Source: CAD feature listing. Evaluate the final solid. Frame: model axes, mm. Give positions to 0.01 mm unless a question says otherwise; leave off trailing zeros. Order: outer loops, then holes, each group sorted by start corner. A loop starts at its lowest first (then second) coordinate and runs counter-clockwise, first axis right, second up. Notation, with made-up numbers: (-31.5, -24) -> (2.5, -24) arc R17 cw to (2.5, -2) -> close; hole circle Ø10 at (2, -25). An arc over 180 degrees is marked (long way). Use CSV: the item, a comma, the result in double quotes.
```python
from build123d import *

# Parameters (mm, degrees)
SKETCH1_W           = 21
SKETCH1_H           = 9
BOSS_EXTRUDE1_DEPTH = 3


with BuildPart() as part:
    # Sketch1 → Boss-Extrude1 (new body)
    with BuildSketch(Plane.XY):
        Polygon((178.5, 24), (181.5, 24), (181.5, 27), (202.5, 27), (202.5, 24), (205.5, 24), (205.5, 27), (210, 27), (210, 28.5), (213, 28.5), (213, 30), (205.5, 30), (205.5, 39), (210, 39), (210, 40.5), (213, 40.5), (213, 42), (6, 42), (6, 40.5), (3, 40.5), (3, 39), (10.5, 39), (10.5, 30), (6, 30), (6, 28.5), (3, 28.5), (3, 27), (10.5, 27), (10.5, 24), (13.5, 24), (13.5, 27), (34.5, 27), (34.5, 24), (37.5, 24), (37.5, 27), (58.5, 27), (58.5, 24), (61.5, 24), (61.5, 27), (82.5, 27), (82.5, 24), (85.5, 24), (85.5, 27), (106.5, 27), (106.5, 24), (109.5, 24), (109.5, 27), (130.5, 27), (130.5, 24), (133.5, 24), (133.5, 27), (154.5, 27), (154.5, 24), (157.5, 24), (157.5, 27), (178.5, 27), align=None)
        with Locations((192, 34.5)):
            Rectangle(SKETCH1_W, SKETCH1_H, mode=Mode.SUBTRACT)
        with Locations((168, 34.5)):
            Rectangle(SKETCH1_W, SKETCH1_H, mode=Mode.SUBTRACT)
        with Locations((144, 34.5)):
            Rectangle(SKETCH1_W, SKETCH1_H, mode=Mode.SUBTRACT)
        with Locations((120, 34.5)):
            Rectangle(SKETCH1_W, SKETCH1_H, mode=Mode.SUBTRACT)
        with Locations((96, 34.5)):
            Rectangle(SKETCH1_W, SKETCH1_H, mode=Mode.SUBTRACT)
        with Locations((72, 34.5)):
            Rectangle(SKETCH1_W, SKETCH1_H, mode=Mode.SUBTRACT)
        with Locations((48, 34.5)):
            Rectangle(SKETCH1_W, SKETCH1_H, mode=Mode.SUBTRACT)
        with Locations((24, 34.5)):
            Rectangle(SKETCH1_W, SKETCH1_H, mode=Mode.SUBTRACT)
    extrude(amount=BOSS_EXTRUDE1_DEPTH)


solid = part.part
```
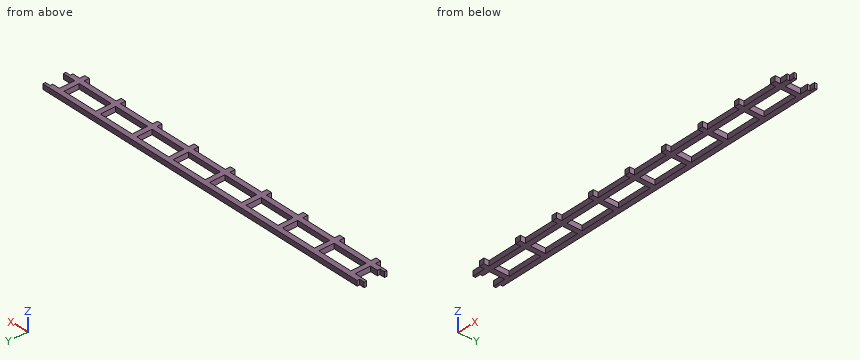
1. Ray query, line 1 along Y through (x, z) = (152, 0.65); line 2 along X through (y, z) = (39.5, 0.95); line 3 along X through (y, z) = (41.25, 2.3). Return the intervals inside material, ascending.
Answer below:
line 1,"y = 27 to 30, 39 to 42"
line 2,"x = 3 to 210"
line 3,"x = 6 to 213"
2. Pin query (flat end, axial travel): P1, Ø0.9, axis at y = 36.5, z = 2, coming from the +X side; P2, Ø1.5, axis at y = 36, z = 1.5, coming from the -X side; P3, Ø1.5, axis at x = 6, z = 2, coming from the -Y side. Return the tip coordinate at first contact, or that it passes through.
Answer below:
P1,"stops at x = 205.5"
P2,"stops at x = 10.5"
P3,"stops at y = 27"
3. Section query B-B on y = 34. Count the separate pieces of the cut face and the enclosed holes in it, plus the area to 3 significant figures.
Answer below:
separate pieces,"9"
enclosed holes,"0"
area,"81.0 mm²"
4. Section query A-A on x = 53. Return loops of the section in (y, z), plus the area to 3 significant figures.
Answer below:
outline,"(27, 0) -> (30, 0) -> (30, 3) -> (27, 3) -> close; (39, 0) -> (42, 0) -> (42, 3) -> (39, 3) -> close"
area,"18.0 mm²"
